Geometry check sheet. Reference: the model listing, model coordinates, mm. Round coordinates to 2 decimals unless told otherwise and drop trailing zeros. Loops run counter-clockwise (first coordinate to the right, second up) from the corner with the lowest first, then second, coordinate; pieces in that order, holes last. Notation, with made-up numbers: M 52.25,34.25 L 69.25,34.25 A15 ccw 69.25,63.25 Z; hole C 77.5,45.25 d3. An arc over 180 degrees is marked long. Answer in a Markdown table with one row per item. Add a question column.
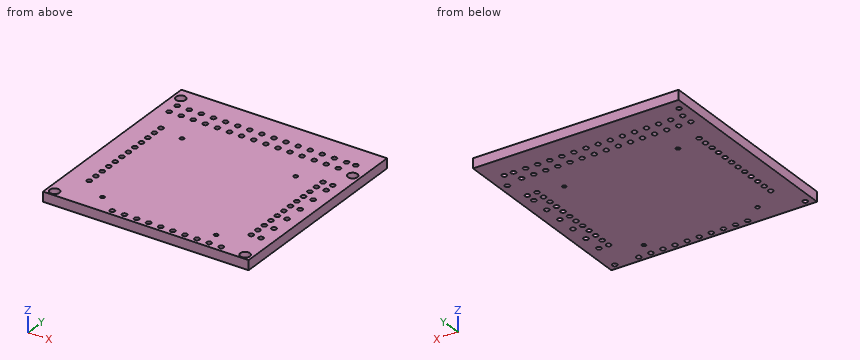
```python
from build123d import *

# Parameters (mm, degrees)
F0_W     = 170
F0_H     = 170
F0_R     = 2
F0_R_2   = 1.65
F1_DEPTH = 8
F2_R     = 4
F2_R_2   = 2
F3_DEPTH = 6


with BuildPart() as f1:
    # F0 (on Top) → F1 (new body)
    with BuildSketch(Plane.XY):
        with Locations((85, -85)):
            Rectangle(F0_W, F0_H)
        with Locations((6.35, -165.1)):
            Circle(F0_R, mode=Mode.SUBTRACT)
        with Locations((18, -139.89)):
            Circle(F0_R, mode=Mode.SUBTRACT)
        with Locations((18, -131.89)):
            Circle(F0_R, mode=Mode.SUBTRACT)
        with Locations((54.2, -165.3)):
            Circle(F0_R, mode=Mode.SUBTRACT)
        with Locations((64.2, -165.3)):
            Circle(F0_R, mode=Mode.SUBTRACT)
        with Locations((74.2, -165.3)):
            Circle(F0_R, mode=Mode.SUBTRACT)
        with Locations((38.01, -153.49)):
            Circle(F0_R_2, mode=Mode.SUBTRACT)
        with Locations((18, -123.89)):
            Circle(F0_R, mode=Mode.SUBTRACT)
        with Locations((18, -115.89)):
            Circle(F0_R, mode=Mode.SUBTRACT)
        with Locations((18, -107.89)):
            Circle(F0_R, mode=Mode.SUBTRACT)
        with Locations((18, -99.89)):
            Circle(F0_R, mode=Mode.SUBTRACT)
        with Locations((18, -91.89)):
            Circle(F0_R, mode=Mode.SUBTRACT)
        with Locations((18, -83.89)):
            Circle(F0_R, mode=Mode.SUBTRACT)
        with Locations((84.2, -165.3)):
            Circle(F0_R, mode=Mode.SUBTRACT)
        with Locations((94.2, -165.3)):
            Circle(F0_R, mode=Mode.SUBTRACT)
        with Locations((104.2, -165.3)):
            Circle(F0_R, mode=Mode.SUBTRACT)
        with Locations((114.2, -165.3)):
            Circle(F0_R, mode=Mode.SUBTRACT)
        with Locations((124.2, -165.3)):
            Circle(F0_R, mode=Mode.SUBTRACT)
        with Locations((134.2, -165.3)):
            Circle(F0_R, mode=Mode.SUBTRACT)
        with Locations((131.99, -153.49)):
            Circle(F0_R_2, mode=Mode.SUBTRACT)
        with Locations((144.2, -165.3)):
            Circle(F0_R, mode=Mode.SUBTRACT)
        with Locations((163.83, -165.1)):
            Circle(F0_R, mode=Mode.SUBTRACT)
        with Locations((152, -139.89)):
            Circle(F0_R, mode=Mode.SUBTRACT)
        with Locations((152, -131.89)):
            Circle(F0_R, mode=Mode.SUBTRACT)
        with Locations((160, -139.89)):
            Circle(F0_R, mode=Mode.SUBTRACT)
        with Locations((152, -123.89)):
            Circle(F0_R, mode=Mode.SUBTRACT)
        with Locations((160, -123.89)):
            Circle(F0_R, mode=Mode.SUBTRACT)
        with Locations((152, -115.89)):
            Circle(F0_R, mode=Mode.SUBTRACT)
        with Locations((152, -107.89)):
            Circle(F0_R, mode=Mode.SUBTRACT)
        with Locations((160, -107.89)):
            Circle(F0_R, mode=Mode.SUBTRACT)
        with Locations((152, -99.89)):
            Circle(F0_R, mode=Mode.SUBTRACT)
        with Locations((152, -91.89)):
            Circle(F0_R, mode=Mode.SUBTRACT)
        with Locations((152, -83.89)):
            Circle(F0_R, mode=Mode.SUBTRACT)
        with Locations((160, -91.89)):
            Circle(F0_R, mode=Mode.SUBTRACT)
        with Locations((18, -75.89)):
            Circle(F0_R, mode=Mode.SUBTRACT)
        with Locations((18, -67.89)):
            Circle(F0_R, mode=Mode.SUBTRACT)
        with Locations((18, -59.89)):
            Circle(F0_R, mode=Mode.SUBTRACT)
        with Locations((18, -51.89)):
            Circle(F0_R, mode=Mode.SUBTRACT)
        with Locations((38.01, -55.7)):
            Circle(F0_R_2, mode=Mode.SUBTRACT)
        with Locations((10, -30)):
            Circle(F0_R, mode=Mode.SUBTRACT)
        with Locations((20, -30)):
            Circle(F0_R, mode=Mode.SUBTRACT)
        with Locations((10, -20)):
            Circle(F0_R, mode=Mode.SUBTRACT)
        with Locations((20, -20)):
            Circle(F0_R, mode=Mode.SUBTRACT)
        with Locations((6.35, -10.16)):
            Circle(F0_R, mode=Mode.SUBTRACT)
        with Locations((30, -30)):
            Circle(F0_R, mode=Mode.SUBTRACT)
        with Locations((30, -20)):
            Circle(F0_R, mode=Mode.SUBTRACT)
        with Locations((40, -30)):
            Circle(F0_R, mode=Mode.SUBTRACT)
        with Locations((50, -30)):
            Circle(F0_R, mode=Mode.SUBTRACT)
        with Locations((40, -20)):
            Circle(F0_R, mode=Mode.SUBTRACT)
        with Locations((50, -20)):
            Circle(F0_R, mode=Mode.SUBTRACT)
        with Locations((60, -30)):
            Circle(F0_R, mode=Mode.SUBTRACT)
        with Locations((60, -20)):
            Circle(F0_R, mode=Mode.SUBTRACT)
        with Locations((70, -30)):
            Circle(F0_R, mode=Mode.SUBTRACT)
        with Locations((80, -30)):
            Circle(F0_R, mode=Mode.SUBTRACT)
        with Locations((70, -20)):
            Circle(F0_R, mode=Mode.SUBTRACT)
        with Locations((80, -20)):
            Circle(F0_R, mode=Mode.SUBTRACT)
        with Locations((131.99, -55.7)):
            Circle(F0_R_2, mode=Mode.SUBTRACT)
        with Locations((152, -75.89)):
            Circle(F0_R, mode=Mode.SUBTRACT)
        with Locations((160, -75.89)):
            Circle(F0_R, mode=Mode.SUBTRACT)
        with Locations((152, -67.89)):
            Circle(F0_R, mode=Mode.SUBTRACT)
        with Locations((152, -59.89)):
            Circle(F0_R, mode=Mode.SUBTRACT)
        with Locations((160, -59.89)):
            Circle(F0_R, mode=Mode.SUBTRACT)
        with Locations((152, -51.89)):
            Circle(F0_R, mode=Mode.SUBTRACT)
        with Locations((160, -51.89)):
            Circle(F0_R, mode=Mode.SUBTRACT)
        with Locations((163.83, -33.02)):
            Circle(F0_R, mode=Mode.SUBTRACT)
        with Locations((90, -30)):
            Circle(F0_R, mode=Mode.SUBTRACT)
        with Locations((90, -20)):
            Circle(F0_R, mode=Mode.SUBTRACT)
        with Locations((100, -30)):
            Circle(F0_R, mode=Mode.SUBTRACT)
        with Locations((110, -30)):
            Circle(F0_R, mode=Mode.SUBTRACT)
        with Locations((100, -20)):
            Circle(F0_R, mode=Mode.SUBTRACT)
        with Locations((110, -20)):
            Circle(F0_R, mode=Mode.SUBTRACT)
        with Locations((120, -30)):
            Circle(F0_R, mode=Mode.SUBTRACT)
        with Locations((120, -20)):
            Circle(F0_R, mode=Mode.SUBTRACT)
        with Locations((130, -30)):
            Circle(F0_R, mode=Mode.SUBTRACT)
        with Locations((130, -20)):
            Circle(F0_R, mode=Mode.SUBTRACT)
        with Locations((140, -30)):
            Circle(F0_R, mode=Mode.SUBTRACT)
        with Locations((150, -30)):
            Circle(F0_R, mode=Mode.SUBTRACT)
        with Locations((140, -20)):
            Circle(F0_R, mode=Mode.SUBTRACT)
        with Locations((150, -20)):
            Circle(F0_R, mode=Mode.SUBTRACT)
        with Locations((157.560000028, -20)):
            Circle(F0_R, mode=Mode.SUBTRACT)
    extrude(amount=F1_DEPTH)

    # F2 (on face) → F3 (cut)
    with BuildSketch(Plane.XY.offset(8)):
        with Locations((163.83, -33.02)):
            Circle(F2_R)
        with Locations((163.83, -33.02)):
            Circle(F2_R_2, mode=Mode.SUBTRACT)
        with Locations((163.83, -165.1)):
            Circle(F2_R)
        with Locations((163.83, -165.1)):
            Circle(F2_R_2, mode=Mode.SUBTRACT)
        with Locations((6.35, -165.1)):
            Circle(F2_R)
        with Locations((6.35, -165.1)):
            Circle(F2_R_2, mode=Mode.SUBTRACT)
        with Locations((6.35, -10.16)):
            Circle(F2_R)
        with Locations((6.35, -10.16)):
            Circle(F2_R_2, mode=Mode.SUBTRACT)
    extrude(amount=-F3_DEPTH, mode=Mode.SUBTRACT)


solid = f1.part
```
1) Cross-section at C-C, the plane y = -123.89. Record the boundary of the cut face in (x, z).
2) Thickness scan on L1, parallel to X at y = -131.5, z = 6; L2, parallel to X at y = -139.89, z = 2.5; L3, parallel to Y at x = 41.5, z = 1.5. Record the ranges inside material, lowest first. Write a range as [from, to].
3) Cross-section at D-D, the plane x = 110. Record the boundary of the cut face in (y, z).
4) Cross-section at A-A, the plane y = -83.89. Record the boundary of the cut face in (x, z), plus the area to 3 significant figures.
5) Go/stop test with flat-tipped pins: pin 1 (3.5 mm diameter, centred on x = 152, y = -107.89, fed in from -Z); pin 2 (2.5 mm diameter, centred on x = 165.5, y = -34, fed in from +Z). Record where each tip stops, or that it passes through.
6) Cross-section at B-B, the plane x = 84.2. Record the boundary of the cut face in (y, z), plus the area to 3 significant figures.
Worked answers:
| question | item | result |
|---|---|---|
| 1 | outline | M 0,0 L 16,0 L 16,8 L 0,8 Z; M 20,0 L 150,0 L 150,8 L 20,8 Z; M 154,0 L 158,0 L 158,8 L 154,8 Z; M 162,0 L 170,0 L 170,8 L 162,8 Z |
| 2 | L1 | x = [0, 16.04], [19.96, 150.04], [153.96, 170] |
| 2 | L2 | x = [0, 16], [20, 150], [154, 158], [162, 170] |
| 2 | L3 | y = [-170, -31.32], [-28.68, -21.32], [-18.68, 0] |
| 3 | outline | M -170,0 L -32,0 L -32,8 L -170,8 Z; M -28,0 L -22,0 L -22,8 L -28,8 Z; M -18,0 L 0,0 L 0,8 L -18,8 Z |
| 4 | outline | M 0,0 L 16,0 L 16,8 L 0,8 Z; M 20,0 L 150,0 L 150,8 L 20,8 Z; M 154,0 L 170,0 L 170,8 L 154,8 Z |
| 4 | area | 1,300 mm2 |
| 5 | pin 1 | passes through |
| 5 | pin 2 | stops at z = 2 |
| 6 | outline | M -170,0 L -167.3,0 L -167.3,8 L -170,8 Z; M -163.3,0 L 0,0 L 0,8 L -163.3,8 Z |
| 6 | area | 1,330 mm2 |
